from build123d import *

# Parameters (mm, degrees)
F1_DEPTH = 4.8


with BuildPart() as f1:
    # F0 (on Top) → F1 (new body)
    with BuildSketch(Plane.XY):
        Polygon((-82.595532, 18.481104), (-87.095532, 18.481104), (-87.095532, -13.960981), (85.034968, -13.960981), (85.034968, -9.460981), (90.034968, -9.460981), (90.034968, 23.481104), (-82.595532, 23.481104), align=None)
        Polygon((85.034968, 60.923189), (-87.095532, 60.923189), (-87.095532, 28.481104), (-82.595532, 28.481104), (-82.595532, 23.481104), (90.034968, 23.481104), (90.034968, 56.423189), (85.034968, 56.423189), align=None)
        Polygon((262.665468, 23.481104), (90.034968, 23.481104), (90.034968, -9.460981), (95.034968, -9.460981), (95.034968, -13.960981), (267.165468, -13.960981), (267.165468, 18.481104), (262.665468, 18.481104), align=None)
        Polygon((267.165468, 60.923189), (95.034968, 60.923189), (95.034968, 56.423189), (90.034968, 56.423189), (90.034968, 23.481104), (262.665468, 23.481104), (262.665468, 28.481104), (267.165468, 28.481104), align=None)
        Polygon((85.034968, -9.460981), (85.034968, -13.960981), (95.034968, -13.960981), (95.034968, -9.460981), (90.034968, -9.460981), align=None)
    extrude(amount=F1_DEPTH)


solid = f1.part
Geometry check sheet. Reference: the model listing, model coordinates, mm. Give positions to 0.01 mm unless a question says otherwise; leave off trailing zeros. Order: outer loops, then holes, each group sorted by start corner. A loop starts at its lowest first (then second) coordinate and runs counter-clockwise, first axis right, second up. Notation, with made-up numbers: M -29.5,-36.75 L 13.5,-36.75 A9 cw 13.5,-28.75 Z; hole C -14,38 d9. An arc over 180 degrees is marked long. Use a Markdown table: item, result.
Item 1: Depth check by flat-ended pin: P1, Ø1, axis at y = 25.5, z = 0.5, coming from the +X side; P2, Ø2.5, axis at y = 26, z = 2.5, coming from the -X side; P3, Ø1.4, axis at x = 90.5, z = 3.5, coming from the +Y side. Enter the tip coordinate at first touch or a pass-through.
Answers follow:
| item | result |
|---|---|
| P1 | stops at x = 262.67 |
| P2 | stops at x = -82.6 |
| P3 | stops at y = 56.42 |
Item 2: Section check A-A (y = 23). Record the cut outline in (x, z).
Answers follow:
| item | result |
|---|---|
| outline | M -82.6,0 L 262.67,0 L 262.67,4.8 L -82.6,4.8 Z |
Item 3: Material ranges on line 1 along X through (y, z) = (58, 4.25); line 2 along X through (y, z) = (22.5, 3.45); line 3 along Y through (x, z) = (90, 1), recorded low to high.
Answers follow:
| item | result |
|---|---|
| line 1 | x = -87.1 to 85.03, 95.03 to 267.17 |
| line 2 | x = -82.6 to 262.67 |
| line 3 | y = -13.96 to 56.42 |
